```python
from build123d import *

# Parameters (mm, degrees)
RESSALTO_EXTRUS_O1_DEPTH = 10
FURO_COM_FOLGA_DE_M61_D  = 6.6


with BuildPart() as part:
    # Esboço1 → Ressalto-extrusão1 (new body)
    with BuildSketch(Plane.XY):
        with BuildLine():
            Line((715.821206727, 0), (900, 0))
            Line((900, 0), (900, 1300))
            Line((900, 1300), (-900, 1300))
            Line((-900, 1300), (-900, 0))
            Line((-900, 0), (-715.821206727, 0))
            ThreePointArc((-715.821206727, 0), (0, 1220), (715.821206727, 0))
        make_face()
    extrude(amount=RESSALTO_EXTRUS_O1_DEPTH)

    # Furo com folga de M61 (through all)
    with Locations(Plane(origin=(0, 400, -6), x_dir=(-1, 0, 0), z_dir=(0, 0, -1))):
        with Locations((0, 851.109495843), (291.096591754, 799.781312724), (547.082638414, 651.987699776), (-291.096591754, 799.781312724), (-547.082638414, 651.987699776)):
            Hole(FURO_COM_FOLGA_DE_M61_D / 2)


solid = part.part
```
Design review of the part built by this model. Coordinates are the model's own, in mm. Give positions to 0.01 mm unless a question says otherwise; leave off trailing zeros. Loops run counter-clockwise (first coordinate to the right, second up) from the corner with the lowest first, then second, coordinate; pieces in that order, holes last. Notation, with made-up numbers: M -38.5,32 L 5.5,32 A15 ccw 5.5,59 Z; hole C 24,68 d8. An arc over 180 degrees is marked long. Return JSON: item names as keys, results as strings. Group by question number.
Item 1: We need section B-B (z = 6.5). Give the boundary of the cut face in (x, y), and give its area (3 significant figures).
Item 2: We need section A-A (y = 400). Give the boundary of the cut face in (x, z).
Item 3: We need section D-D (x = 689). Give the boundary of the cut face in (y, z).
Item 4: Mouldability with a two-part tool opening along X and no side actions: class faces 1 (the cylindrical face through (-23.879, 1219.652, 4.93)), 2 (the flat face through (-4, 1231, 0)) as released by +X, released by -X, zero draft, split by the parting line, or undercut.
Item 5: Insertion check: pin 1 Ø5 at (x, z) = (340.5, 4.5) entering from -Y; pin 2 Ø3 at (x, z) = (458, 7.5) entering from -Y; pin 3 Ø6 at (x, y) = (0, 1251.11) entering from +Z; pin 4 Ø2 at (x, z) = (683.5, 6.5) entering from -Y. Each pin has a flat end and moves straight along its axis. Give the tip position at first contact, or say it passes through.
Item 6: We need section C-C (y = 699). Give the boundary of the cut face in (x, z), and give its area (3 significant figures).
Item 7: For probe 1 along X at (y, z) = (391, 7.25); probe 2 along Y at (x, z) = (0, 7.5); probe 3 along X at (y, z) = (412.5, 2.5), list the stretches that pass through material, from the lowest coordinate up.
Output:
{
 "1": {"outline": "M -900,0 L -715.82,0 A820 cw long 715.82,0 L 900,0 L 900,1300 L -900,1300 Z; hole C -547.08,1051.99 d6.6; hole C -291.1,1199.78 d6.6; hole C 0,1251.11 d6.6; hole C 291.1,1199.78 d6.6; hole C 547.08,1051.99 d6.6", "area": "655,000 mm^2"},
 "2": {"outline": "M -900,0 L -820,0 L -820,10 L -900,10 Z; M 820,0 L 900,0 L 900,10 L 820,10 Z"},
 "3": {"outline": "M 844.61,0 L 1300,0 L 1300,10 L 844.61,10 Z"},
 "4": {"face 1": "undercut", "face 2": "zero draft"},
 "5": {"pin 1": "stops at y = 1144.82", "pin 2": "stops at y = 1079.16", "pin 3": "passes through", "pin 4": "stops at y = 851.51"},
 "6": {"outline": "M -900,0 L -763.54,0 L -763.54,10 L -900,10 Z; M 763.54,0 L 900,0 L 900,10 L 763.54,10 Z", "area": "2,730 mm^2"},
 "7": {"probe 1": "x = -900 to -819.95, 819.95 to 900", "probe 2": "y = 1220 to 1247.81, 1254.41 to 1300", "probe 3": "x = -900 to -819.9, 819.9 to 900"}
}
